from build123d import *

# Parameters (mm, degrees)
SKETCH_1_W          = 62
SKETCH_1_H          = 45
EXTRUDE_1_DEPTH     = 30
SKETCH_2_R          = 16.5
EXTRUDE_2_DEPTH     = 52
SKETCH_4_W          = 40
SKETCH_4_H          = 39
EXTRUDE_4_DEPTH     = 20
CUT_EXTRUDE_1_REACH = 144.518
SKETCH_8_R          = 5
SKETCH_8_R_2        = 2
EXTRUDE_6_DEPTH     = 4.5
SKETCH_8_3_R        = 6
EXTRUDE_7_DEPTH     = 4.5
SKETCH_9_R          = 4
CUT_EXTRUDE_2_DEPTH = 10


with BuildPart() as part:
    # Sketch 1 → Extrude 1 (new body)
    with BuildSketch(Plane.XY.offset(10)):
        Rectangle(SKETCH_1_W, SKETCH_1_H)
    extrude(amount=EXTRUDE_1_DEPTH)

    # Sketch 2 → Extrude 2 (add)
    with BuildSketch(Plane(origin=(31, 0, 0), x_dir=(0, 0, -1), z_dir=(1, 0, 0))):
        with Locations(Location((-25, 0, 0), (0, 0, 155.380022671))):
            Circle(SKETCH_2_R)
    extrude(amount=EXTRUDE_2_DEPTH)

    # Sketch 4 → Extrude 4 (add)
    with BuildSketch(Plane(origin=(83, 0, 0), x_dir=(0, 0, -1), z_dir=(1, 0, 0))):
        with Locations((-23, 0)):
            Rectangle(SKETCH_4_W, SKETCH_4_H)
    extrude(amount=EXTRUDE_4_DEPTH)

    # Sketch 6 → Cut-Extrude 1 (cut, up to next)
    with BuildSketch(Plane(origin=(103, 0, 0), x_dir=(0, 0, -1), z_dir=(1, 0, 0)), mode=Mode.PRIVATE) as cut_extrude_1_sk1:
        with BuildLine():
            Line((-43, 19.5), (-43, -0.5))
            ThreePointArc((-43, -0.5), (-37.142135635, 13.642135613), (-23.000000031, 19.5))
            Line((-23.000000031, 19.5), (-43, 19.5))
        make_face()
    cut_extrude_1_tool1 = extrude(cut_extrude_1_sk1.sketch, amount=-CUT_EXTRUDE_1_REACH, mode=Mode.PRIVATE) & part.part
    # Sketch 6 → Cut-Extrude 1 (cut, up to next)
    with BuildSketch(Plane(origin=(103, 0, 0), x_dir=(0, 0, -1), z_dir=(1, 0, 0)), mode=Mode.PRIVATE) as cut_extrude_1_sk2:
        with BuildLine():
            Line((-3, 19.5), (-23.000000031, 19.5))
            ThreePointArc((-23.000000031, 19.5), (-8.857864387, 13.642135635), (-3, -0.5))
            Line((-3, -0.5), (-3, 19.5))
        make_face()
    cut_extrude_1_tool2 = extrude(cut_extrude_1_sk2.sketch, amount=-CUT_EXTRUDE_1_REACH, mode=Mode.PRIVATE) & part.part
    add(cut_extrude_1_tool1.solids().sort_by_distance((103, 15.032641, 38.532641))[0], mode=Mode.SUBTRACT)
    add(cut_extrude_1_tool2.solids().sort_by_distance((103, 15.032641, 7.467359))[0], mode=Mode.SUBTRACT)

    # Sketch 8 → Extrude 6 (add)
    # profile 1 of 6: a face of its own
    with BuildSketch(Plane(origin=(0, 0, 10), x_dir=(-1, 0, 0), z_dir=(0, 0, -1))):
        with Locations(Location((0.5, -15, 0), (0, 0, 180))):
            Circle(SKETCH_8_R)
        with Locations((0.5, -15)):
            Circle(SKETCH_8_R_2, mode=Mode.SUBTRACT)
    # profile 2 of 6: a face of its own
    with BuildSketch(Plane(origin=(0, 0, 10), x_dir=(-1, 0, 0), z_dir=(0, 0, -1))):
        with Locations(Location((-19.5, -15, 0), (0, 0, 180))):
            Circle(SKETCH_8_R)
        with Locations((-19.5, -15)):
            Circle(SKETCH_8_R_2, mode=Mode.SUBTRACT)
    # profile 3 of 6: a face of its own
    with BuildSketch(Plane(origin=(0, 0, 10), x_dir=(-1, 0, 0), z_dir=(0, 0, -1))):
        with Locations(Location((20.5, -15, 0), (0, 0, 180))):
            Circle(SKETCH_8_R)
        with Locations((20.5, -15)):
            Circle(SKETCH_8_R_2, mode=Mode.SUBTRACT)
    # profile 4 of 6: a face of its own
    with BuildSketch(Plane(origin=(0, 0, 10), x_dir=(-1, 0, 0), z_dir=(0, 0, -1))):
        with Locations(Location((20.5, 15, 0), (0, 0, 180))):
            Circle(SKETCH_8_R)
        with Locations((20.5, 15)):
            Circle(SKETCH_8_R_2, mode=Mode.SUBTRACT)
    # profile 5 of 6: a face of its own
    with BuildSketch(Plane(origin=(0, 0, 10), x_dir=(-1, 0, 0), z_dir=(0, 0, -1))):
        with Locations(Location((0.5, 15, 0), (0, 0, 180))):
            Circle(SKETCH_8_R)
        with Locations((0.5, 15)):
            Circle(SKETCH_8_R_2, mode=Mode.SUBTRACT)
    # profile 6 of 6: a face of its own
    with BuildSketch(Plane(origin=(0, 0, 10), x_dir=(-1, 0, 0), z_dir=(0, 0, -1))):
        with Locations(Location((-19.5, 15, 0), (0, 0, 180))):
            Circle(SKETCH_8_R)
        with Locations((-19.5, 15)):
            Circle(SKETCH_8_R_2, mode=Mode.SUBTRACT)
    extrude_6 = extrude(amount=EXTRUDE_6_DEPTH)

    # Mirror 1: Extrude 6 across plane
    add(extrude_6.mirror(Plane(origin=(0, 0, 25), x_dir=(1, 0, 0), z_dir=(0, 0, -1))))

    # Sketch 8_3 → Extrude 7 (add)
    with BuildSketch(Plane(origin=(0, 0, 10), x_dir=(-1, 0, 0), z_dir=(0, 0, -1))):
        with Locations(Location((12.5, 0, 0), (0, 0, 180))):
            Circle(SKETCH_8_3_R)
    extrude(amount=EXTRUDE_7_DEPTH)

    # Sketch 9 → Cut-Extrude 2 (cut)
    with BuildSketch(Plane(origin=(0, 0, 5.5), x_dir=(-1, 0, 0), z_dir=(0, 0, -1))):
        with Locations((12.5, 0)):
            Circle(SKETCH_9_R)
    extrude(amount=-CUT_EXTRUDE_2_DEPTH, mode=Mode.SUBTRACT)


solid = part.part
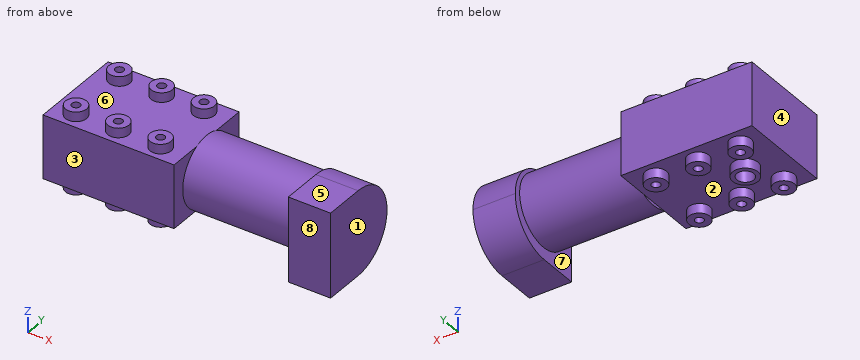
Read the model definition and answer for the solid it produces. Units are mm, in the model's axes. Face numbers are marked on the shaded views. A direction names the side the tool comes from. Round coordinates to 2 decimals unless told otherwise and drop trailing zeros. Order: outer loops, then holes, each group sorted by start corner. A loop starts at its lowest first (then second) coordinate and runs counter-clockwise, first axis right, second up. Notation, with made-up numbers: (89.25, 64.25) - (100.25, 64.25) arc R9 ccw to (100.25, 80.25) - close; hole circle Ø2 at (76.25, 9.5). An arc over 180 degrees is marked (long way). Use one line per item in the form item = value. Start each with the question number.
(1) Determine the mould class of the marked faces 1, 2 and 3 for opening direction X: +X half, -X half, draft (parallel to the pull), parting line (faces both ways), or undercut.
(2) The part is cut by section C-C (y = -2). Give the vertices of the cut face in (x, z), then the cut area to 3 significant figures.
(3) The part is cut by section D-D (x = 49.5). Give the vertices of the cut face in (y, z), then the cut area to 3 significant figures.
(4) Flat-ended cylindrical pins translate along their axes: pin 1 Ø6 at (x, y) = (-15.5, 0) entering from -Z; pin 2 Ø7 at (x, y) = (-12.5, 0) entering from -Z; pin 3 Ø2 at (x, y) = (71.5, 8.5) entering from +Z. Find the tip coordinate at first contact, or state that the pin passes through.
(5) The part is cut by section B-B (z = 38.5). Give the vertices of the cut face in (x, y).
(6) The part is cut by section A-A (x = -12.5). Give the vertices of the cut face in (y, z), then the cut area to 3 significant figures.
(7) Find the intervals of material crossed by line 1 along Y through (x, z) = (-0.5, 7.8); line 2 along Y through (x, z) = (-12.5, 13.75); line 3 along Y through (x, z) = (19, 43), in increasing order. Write a range as from..to.
(8) For the marked faces 4, 5, 6, 7 and 8, determine the directions among +Z, -Z, +X, -X, +Y, -Y from which every point of the face is accessible in a straight line to the end or side of a thin tool.
Checked values:
q1.face_1 = +X half
q1.face_2 = undercut
q1.face_3 = draft
q2.outline = (-31, 10) - (-18.16, 10) - (-18.16, 5.5) - (-15.96, 5.5) - (-15.96, 15.5) - (-9.04, 15.5) - (-9.04, 5.5) - (-6.84, 5.5) - (-6.84, 10) - (31, 10) - (31, 8.62) - (83, 8.62) - (83, 3) - (103, 3) - (103, 43) - (83, 43) - (83, 41.38) - (31, 41.38) - (31, 40) - (-31, 40) - close
q2.area = 4,340 mm^2
q3.outline = circle Ø33 at (0, 25)
q3.area = 855 mm^2
q4.pin_1 = 5.5
q4.pin_2 = 15.5
q4.pin_3 = 39.7
q5.outline = (-31, -22.5) - (31, -22.5) - (31, -9.49) - (83, -9.49) - (83, -19.5) - (103, -19.5) - (103, 12.14) - (83, 12.14) - (83, 9.49) - (31, 9.49) - (31, 22.5) - (-31, 22.5) - close
q6.outline = (-22.5, 10) - (-6, 10) - (-6, 5.5) - (-4, 5.5) - (-4, 15.5) - (4, 15.5) - (4, 5.5) - (6, 5.5) - (6, 10) - (22.5, 10) - (22.5, 40) - (-22.5, 40) - close
q6.area = 1,320 mm^2
q7.line_1 = -20..-17, -13..-10, 10..13, 17..20
q7.line_2 = -22.5..-4, 4..22.5
q7.line_3 = -19.97..-16.94, -13.06..-10.03, 10.03..13.06, 16.94..19.97
q8.face_4 = +Z, -Z, -X, +Y, -Y
q8.face_5 = +Z, +X, +Y, -Y
q8.face_6 = +Z
q8.face_7 = none
q8.face_8 = +Z, -Z, +X, -Y
